from build123d import *

# Parameters (mm, degrees)
F0_W     = 15
F0_H     = 15
F1_DEPTH = 15
F3_DEPTH = 15


with BuildPart() as f1:
    # F0 (on Top) → F1 (new body)
    with BuildSketch(Plane.XY):
        with Locations((7.5, -7.5)):
            Rectangle(F0_W, F0_H)
    extrude(amount=F1_DEPTH)

    # F2 (on face) → F3 (join)
    with BuildSketch(Plane.XZ.offset(15)):
        Polygon((7.5, 22.5), (0, 15), (15, 15), align=None)
    extrude(amount=-F3_DEPTH)


solid = f1.part
The listing builds one solid part. Answer for the finished solid, in the listing's coordinates (mm). Round coordinates to 2 decimals unless told otherwise and drop trailing zeros. Order: outer loops, then holes, each group sorted by start corner. A loop starts at its lowest first (then second) coordinate and runs counter-clockwise, first axis right, second up. Notation, with made-up numbers: (30.25, -14.5) -> (86.25, -14.5) arc R22 ccw to (86.25, -1.5) -> close; hole circle Ø7 at (12.5, -15). An arc over 180 degrees is marked (long way). One line per item, written item: value.
Item 1: Find section A-A, the plane y = -3.75. Give the vertices of the cut face in (x, z).
Taken from the geometry:
outline: (0, 0) -> (15, 0) -> (15, 15) -> (7.5, 22.5) -> (0, 15) -> close
Item 2: Find section C-C, the plane x = 5. Give the vertices of the cut face in (y, z).
Taken from the geometry:
outline: (-15, 0) -> (0, 0) -> (0, 20) -> (-15, 20) -> close
Item 3: Given P1, Ø1, axis at y = -3, z = 18.5, coming from the +X side, flat-ended and moving along its own axis, determine where the tip first touches the part or whether it passes through.
Taken from the geometry:
P1: stops at x = 12
Item 4: Straight lines are drawn through the part: L1, parallel to Z at x = 1.5, y = -11.75; L2, parallel to X at y = -0.75, z = 17; L3, parallel to Z at x = 12.5, y = -5.5. For each, find the intervals that lie inside material, in ascending order.
Taken from the geometry:
L1: z = 0 to 16.5
L2: x = 2 to 13
L3: z = 0 to 17.5
Item 5: Find section B-B, the plane z = 19.75. Give the vertices of the cut face in (x, y), then the cut area to 3 significant figures.
Taken from the geometry:
outline: (4.75, -15) -> (10.25, -15) -> (10.25, 0) -> (4.75, 0) -> close
area: 82.5 mm2
